from build123d import *

# Parameters (mm, degrees)
SKETCH1_R           = 5.207
SKETCH1_R_2         = 3.556
BOSS_EXTRUDE1_DEPTH = 1.5875
SKETCH2_R           = 3.175
CUT_EXTRUDE1_DEPTH  = 2.5875
SKETCH3_R           = 4.7625
CUT_EXTRUDE2_DEPTH  = 2.54


with BuildPart() as part:
    # Sketch1 → Boss-Extrude1 (new body)
    with BuildSketch(Plane(origin=(0, 0, 0), x_dir=(1, 0, 0), z_dir=(0, 1, 0))):
        Polygon((-28.60675, 81.407), (28.60675, 81.407), (28.60675, -81.407), (28.60675, -83.693), (-28.60675, -83.693), (-28.60675, -81.407), align=None)
        with Locations((-19.08175, 56.007)):
            Circle(SKETCH1_R, mode=Mode.SUBTRACT)
        with Locations((-19.08175, -56.007)):
            Circle(SKETCH1_R, mode=Mode.SUBTRACT)
        with Locations((13.62075, 68.707)):
            Circle(SKETCH1_R_2, mode=Mode.SUBTRACT)
        with Locations((13.62075, 43.307)):
            Circle(SKETCH1_R_2, mode=Mode.SUBTRACT)
        with Locations((13.62075, -43.307)):
            Circle(SKETCH1_R_2, mode=Mode.SUBTRACT)
        with Locations((13.62075, -68.707)):
            Circle(SKETCH1_R_2, mode=Mode.SUBTRACT)
    extrude(amount=BOSS_EXTRUDE1_DEPTH)

    # Sketch2 → Cut-Extrude1 (cut, through all)
    with BuildSketch(Plane(origin=(0, 1.5875, 0), x_dir=(1, 0, 0), z_dir=(0, 1, 0))):
        with Locations((-16.849815709, 0.01058698)):
            Circle(SKETCH2_R)
    extrude(amount=-CUT_EXTRUDE1_DEPTH, mode=Mode.SUBTRACT)

    # Sketch3 → Cut-Extrude2 (cut)
    with BuildSketch(Plane(origin=(0, 1.5875, 0), x_dir=(1, 0, 0), z_dir=(0, 1, 0))):
        with Locations((15.14475, -1.143)):
            Circle(SKETCH3_R)
    extrude(amount=-CUT_EXTRUDE2_DEPTH, mode=Mode.SUBTRACT)


solid = part.part
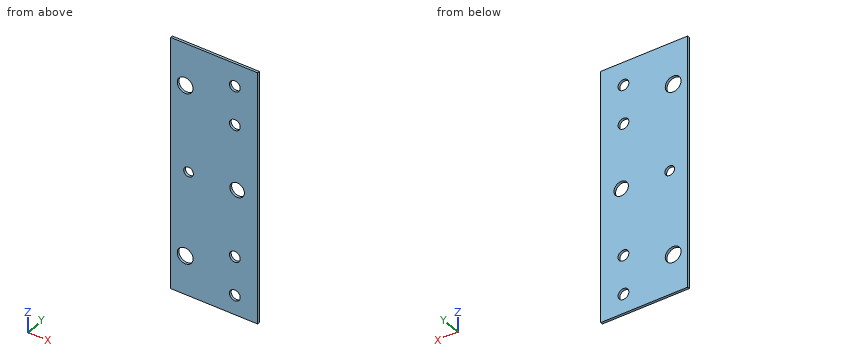
Work out the finished part from the listing and answer in its coordinate system (mm). Round coordinates to 2 decimals unless told otherwise and drop trailing zeros. Loops run counter-clockwise (first coordinate to the right, second up) from the corner with the lowest first, then second, coordinate; pieces in that order, holes last. Notation, with made-up numbers: (17.5, 85) - (66.5, 85) arc R20 cw to (66.5, 100) - close; hole circle Ø11 at (37, 77). An arc over 180 degrees is marked (long way). One line per item, written item: value.
Q1. Find section B-B on z = 54.5. Give the vertices of the cut face in (x, y), and give its area (3 significant figures).
Check values:
outline: (-28.61, 0) - (-24.07, 0) - (-24.07, 1.59) - (-28.61, 1.59) - close; (-14.1, 0) - (28.61, 0) - (28.61, 1.59) - (-14.1, 1.59) - close
area: 75.0 mm2
Q2. Find section C-C on y = 1.05. State how many separate pieces and enclosed holes the cut face has, and give its area (3 significant figures).
Check values:
separate pieces: 1
enclosed holes: 8
area: 9,010 mm2
Q3. Straight lines are drawn through the part: probe 1 along Z at (x, y) = (16, 0.8); probe 2 along Z at (x, y) = (11, 0.95); probe 3 along X at (y, z) = (0.9, 1.5). For each, find the intervals that lie inside material, in ascending order.
Check values:
probe 1: -81.41 to -71.35, -66.06 to -45.95, -40.66 to -3.54, 5.83 to 40.66, 45.95 to 66.06, 71.35 to 83.69
probe 2: -81.41 to -71.11, -66.3 to -45.71, -40.9 to -1.2, 3.49 to 40.9, 45.71 to 66.3, 71.11 to 83.69
probe 3: -28.61 to -19.64, -14.06 to 10.4, 19.89 to 28.61
Q4. Find section A-A on x = -16.5. Give the vertices of the cut face in (y, z).
Check values:
outline: (0, -81.41) - (1.59, -81.41) - (1.59, -60.53) - (0, -60.53) - close; (0, -51.49) - (1.59, -51.49) - (1.59, -3.17) - (0, -3.17) - close; (0, 3.15) - (1.59, 3.15) - (1.59, 51.49) - (0, 51.49) - close; (0, 60.53) - (1.59, 60.53) - (1.59, 83.69) - (0, 83.69) - close
